Geometry: final body of the model. Coordinates: model frame, mm. A direction names the side the tool comes from. Give positions to 0.01 mm unless a question says otherwise; leave off trailing zeros. Write each loop counter-clockwise with the first axis right and the second up, starting at its lowest first coordinate (ties: lowest second). Pieces come first, ordered by that corner, then holes.
from build123d import *

# Parameters (mm, degrees)
FASE1_SIZE                      = 0.8
SCHNITT_LINEAR_AUSTRAGEN1_DEPTH = 10
SCHNITT_LINEAR_START            = -5
SCHNITT_LINEAR_AUSTRAGEN2_DEPTH = 5
FASE2_SIZE                      = 5
VERRUNDUNG1_R                   = 1


# Read off the part's stored shape, not the designer's step: Schnitt-Linear austragen2
with BuildPart() as part:
    # Skizze3 → Rotation1 (revolve)
    with BuildSketch(Plane(origin=(0, 0, 0), x_dir=(0, 0, -1), z_dir=(1, 0, 0)), mode=Mode.PRIVATE) as rotation1_sk:
        Polygon((0, 27.5), (0, 34.9), (6, 34.9), (6, 38.1), (4, 38.1), (4, 42.5), (8, 42.5), (8, 27.5), align=None)
    revolve(rotation1_sk.sketch.rotate(Axis((0, 0, 28.082191781), (0, 0, -1)), 90), axis=Axis((0, 0, 28.082191781), (0, 0, -1)))

    # Fase1
    fase1_edges = [part.edges().sort_by_distance(p)[0] for p in [
        (-27.5, 0, -8),
        (-42.5, 0, -8),
        (-42.5, 0, -4),
        (-38.1, 0, -4),
    ]]
    chamfer(fase1_edges, length=FASE1_SIZE)

    # Skizze4 → Schnitt-Linear austragen1 (cut)
    with BuildSketch(Plane.XY):
        with BuildLine():
            Line((25.617376915, 20), (-25.617376915, 20))
            ThreePointArc((-25.617376915, 20), (-30.731211738, 10.575567367), (-32.5, 0))
            Line((-32.5, 0), (32.5, 0))
            ThreePointArc((32.5, 0), (30.731211738, 10.575567367), (25.617376915, 20))
        make_face()
        with BuildLine():
            Line((32.5, 0), (-32.5, 0))
            ThreePointArc((-32.5, 0), (-30.731211738, -10.575567367), (-25.617376915, -20))
            Line((-25.617376915, -20), (25.617376915, -20))
            ThreePointArc((25.617376915, -20), (30.731211738, -10.575567367), (32.5, 0))
        make_face()
    extrude(amount=-SCHNITT_LINEAR_AUSTRAGEN1_DEPTH, mode=Mode.SUBTRACT)

    # Schnitt-Linear austragen2 outline → Schnitt-Linear austragen2 (cut)
    with BuildSketch(Plane(origin=(0, 0, -8), x_dir=(-1, 0, 0), z_dir=(0, 0, -1)).offset(SCHNITT_LINEAR_START)):
        with BuildLine():
            Line((-20, -20), (-20, -25.617376915))
            ThreePointArc((-20, -25.617376915), (0, -32.5), (20, -25.617376915))
            Line((20, -25.617376915), (20, -20))
            Line((20, -20), (18.874586088, -20))
            ThreePointArc((18.874586088, -20), (0, -27.5), (-18.874586088, -20))
            Line((-18.874586088, -20), (-20, -20))
        make_face()
        with BuildLine():
            Line((20, 20), (20, 25.617376915))
            ThreePointArc((20, 25.617376915), (0, 32.5), (-20, 25.617376915))
            Line((-20, 25.617376915), (-20, 20))
            Line((-20, 20), (-18.874586088, 20))
            ThreePointArc((-18.874586088, 20), (0, 27.5), (18.874586088, 20))
            Line((18.874586088, 20), (20, 20))
        make_face()
    extrude(amount=SCHNITT_LINEAR_AUSTRAGEN2_DEPTH, mode=Mode.SUBTRACT)

    # Fase2
    fase2_edges = [part.edges().sort_by_distance(p)[0] for p in [
        (0, -32.5, -3),
        (0, 32.5, -3),
    ]]
    chamfer(fase2_edges, length=FASE2_SIZE - 0.0001)  # a hair under: the kernel refuses the full size

    # Verrundung1
    verrundung1_edges = [part.edges().sort_by_distance(p)[0] for p in [
        (-34.9, 0, 0),
    ]]
    fillet(verrundung1_edges, radius=VERRUNDUNG1_R)


solid = part.part
Q1. Ray query, line 1 along Y through (x, z) = (0, -5.65); line 2 along Z through (x, y) = (-5, -35); line 3 along X through (y, z) = (-8, -4.75). Return the intervals inside material, ascending.
Filled sheet:
line 1: y = -42.5 to -38.1, -34.9 to -30.15, 30.15 to 34.9, 38.1 to 42.5
line 2: z = -8 to -6
line 3: x = -41.69 to -37.3, -33.97 to -31.5, 31.5 to 33.97, 37.3 to 41.69
Q2. Pull-direction query (Y, two-part tool) for faces 5 (the conical face through (-0.3, 28.4, -3.9)), 6 (the flat face through (-37, -13, -4)); classes: released by +Y, released by -Y, zero draft, split by the parting line, or undercut.
Filled sheet:
face 5: undercut
face 6: zero draft
Q3. Pin query (flat end, axial travel): P1, Ø1.3, axis at y = -22, z = -6.5, coming from the -X side; P2, Ø3.5, axis at y = -22, z = -6.5, coming from the +X side; P3, Ø3.5, axis at x = 21.5, z = -3, coming from the +Y side. Return the tip coordinate at first contact, or that it passes through.
Filled sheet:
P1: stops at x = -36.75
P2: stops at x = 37.37
P3: stops at y = 36.84
Q4. Access query for faces 1 (the flat face through (0, -28, 0)), 2 (the cylindrical face through (-7.57, 34.07, -3.54)), 3 (the flat face through (-22, 20, -4)), 4 (the conical face through (0.3, -28.4, -3.9)). Directions: +Z, -Z, +X, -X, +Y, -Y. A direction counts if a zero-diameter tool reaches every point of the face in a straight line with its end or side. Return the directions, or none.
Filled sheet:
face 1: +Z, +X, -X, +Y, -Y
face 2: +Z
face 3: +Z, -Z
face 4: -Z
Q5. Section A-A on z = -2. Output: boundary loops of the cut face in (x, y), plus the area to 3 significant figures.
Filled sheet:
outline: circle Ø69.8 at (0, 0); hole (-25.62, -20) - (-18.87, -20) arc R27.5 ccw to (18.87, -20) - (25.62, -20) arc R32.5 ccw to (25.62, 20) - (18.87, 20) arc R27.5 ccw to (-18.87, 20) - (-25.62, 20) arc R32.5 ccw to start
area: 1,010 mm2
